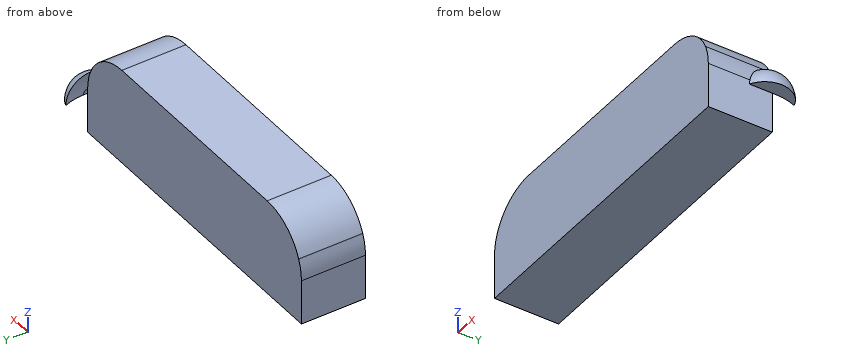
from build123d import *

# Parameters (mm, degrees)
F3_DEPTH      = 25.4
F4_ANGLE_BACK = 90
F4_ANGLE      = 180


with BuildPart() as f3:
    # F2 (on offset) → F3 (new body)
    with BuildSketch(Plane.XZ.offset(25.4)):
        with BuildLine():
            Line((111.518352419, 2.54), (111.518352419, 17.78))
            ThreePointArc((111.518352419, 17.78), (111.1052602487, 21.8564470631), (109.8827795196, 25.7671511769))
            ThreePointArc((109.8827795196, 25.7671511769), (102.3921785764, 34.7387928803), (91.198352419, 38.1))
            Line((91.198352419, 38.1), (4.838352419, 38.1))
            ThreePointArc((4.838352419, 38.1), (-6.3554737384, 34.7387928803), (-13.8460746816, 25.7671511769))
            ThreePointArc((-13.8460746816, 25.7671511769), (-15.0685554108, 21.8564470631), (-15.481647581, 17.78))
            Line((-15.481647581, 17.78), (-15.481647581, 16.035139312))
            Line((-15.481647581, 16.035139312), (-15.481647581, 0))
            Line((-15.481647581, 0), (111.518352419, 0))
            Line((111.518352419, 0), (111.518352419, 2.54))
        make_face()
    extrude(amount=-F3_DEPTH)

    # F0 (on Front) → F4 (revolve)
    with BuildSketch(Plane.XZ, mode=Mode.PRIVATE) as f4_sk:
        with BuildLine():
            ThreePointArc((117.1249815379, 16.035139312), (115.1157614851, 22.1006472259), (109.8827795196, 25.7671511769))
            ThreePointArc((109.8827795196, 25.7671511769), (111.1052602487, 21.8564470631), (111.518352419, 17.78))
            Line((111.518352419, 17.78), (111.518352419, 16.035139312))
            Line((111.518352419, 16.035139312), (117.1249815379, 16.035139312))
        make_face()
    revolve(f4_sk.sketch.rotate(Axis((114.3216669785, 0, 16.035139312), (-1, 0, 0)), -F4_ANGLE_BACK), axis=Axis((114.3216669785, 0, 16.035139312), (-1, 0, 0)), revolution_arc=F4_ANGLE)


solid = f3.part
Geometry check sheet. Reference: the model listing, model coordinates, mm. Coordinates: 2 decimals unless noted, no trailing zeros. Order: outer loops, then holes, each group sorted by start corner. A loop starts at its lowest first (then second) coordinate and runs counter-clockwise, first axis right, second up. Notation, with made-up numbers: (60.5, 24) - (66.5, 24) arc R24 ccw to (66.5, 59) - close; hole circle Ø4 at (84.5, 48.25). An arc over 180 degrees is marked (long way). Answer in a Markdown table with one row per item. Add a question column.
1) Cross-section at D-D, the plane y = -11. Record the cut outline in (x, z), then the cut area to 3 significant figures.
2) Cross-section at C-C, the plane z = 4.5. Record the cut outline in (x, y).
3) Gauge pin test, flat ends, axial feed: P1, Ø14, axis at y = -9.5, z = 5, coming from the +X side; P2, Ø19, axis at x = 41, z = 16, coming from the +Y side; P3, Ø2, axis at y = 4.5, z = 18, coming from the -X side; P4, Ø6, axis at x = 94, y = 0.5, coming from the +Z side. Record the tip position at first contact, or that the pin passes through.
4) Cross-section at A-A, the plane y = -3.5. Record the cut outline in (x, z), then the cut area to 3 significant figures.
5) Cross-section at B-B, the plane x = 45. Record the cut outline in (y, z).
6) Material ranges on line 1 along X through (y, z) = (-6, 7); line 2 along Y through (x, z) = (7, 15.5); line 3 along X through (y, z) = (3.5, 21.5), recorded low to high. Write a range as [from, to].
Check result:
| question | item | result |
|---|---|---|
| 1 | outline | (-15.48, 0) - (111.52, 0) - (111.52, 17.78) arc R20.32 ccw to (91.2, 38.1) - (4.84, 38.1) arc R20.32 ccw to (-15.48, 17.78) - close |
| 1 | area | 4,660 mm² |
| 2 | outline | (-15.48, -25.4) - (111.52, -25.4) - (111.52, 0) - (-15.48, 0) - close |
| 3 | P1 | stops at x = 111.52 |
| 3 | P2 | stops at y = 0 |
| 3 | P3 | stops at x = 111.09 |
| 3 | P4 | stops at z = 38.1 |
| 4 | outline | (-15.48, 0) - (111.52, 0) - (111.52, 16.04) - (116.5, 16.04) arc R9.54 ccw to (110.19, 25.01) arc R20.32 ccw to (91.2, 38.1) - (4.84, 38.1) arc R20.32 ccw to (-15.48, 17.78) - close |
| 4 | area | 4,690 mm² |
| 5 | outline | (-25.4, 0) - (0, 0) - (0, 38.1) - (-25.4, 38.1) - close |
| 6 | line 1 | x = [-15.48, 111.52] |
| 6 | line 2 | y = [-25.4, 0] |
| 6 | line 3 | x = [110.96, 114.78] |
